Source: CAD feature listing. Evaluate the final solid. Frame: model axes, mm. A direction names the side the tool comes from. Give positions to 0.01 mm unless a question says otherwise; leave off trailing zeros. Order: outer loops, then holes, each group sorted by start corner. A loop starts at its lowest first (then second) coordinate and runs counter-clockwise, first axis right, second up. Notation, with made-up numbers: M -13,-9 L 3,-9 A23 cw 3,22 Z; hole C 62.25,-0.5 d5. An arc over 180 degrees is marked long. Answer as a JSON object with one key per item and string values. Group by question number.
1. Section query A-A (y = 76). Output: boundary loops of the cut face in (x, z).
2. Pin query (flat end, axial travel): P1, Ø10, axis at x = 19.05, z = -224.79, coming from the +Y side. Return the tip coordinate at first contact, or that it passes through.
3. Set-up query: faces 5 (the flat face through (38.1, 44, -222)), 6 (the flat face through (19, 44.45, -225)). Return all of +Z, -Z, +X, -X, +Y, -Y with unobstructed straight access to the full face (end or side cutting, diameter ignored); none if empty.
4. Section query B-B (x = 9.5). Output: boundary loops of the cut face in (y, z).
5. Section query C-C (z = -232.5). Output: boundary loops of the cut face in (x, y).
6. Pull-direction query (Z, two-part tool) for faces 1 (the flat face through (23, 0, -228)), 2 (the flat face through (19, 44, 0)), 3 (the flat face through (19, 67, -243.84)), 4 (the flat face through (19, 67, -205.74)); classes: +Z half, -Z half, draft (parallel to the pull), parting line (faces both ways), or undercut.
7. Material intervals for L1, parallel to X at y = 4.25, z = -224.79 (3 decimals); L2, parallel to Z at x = 16, y = 47; L3, parallel to Z at x = 19.05, y = 6.5 (3 decimals), sorted ascending. Write a range as [from, to].
Autodesk Inventor part; units mm, degrees
ref_plane "YZ Plane" through (0, 0, 0) normal (1, 0, 0) x (0, 1, 0)
ref_plane "XZ Plane" through (0, 0, 0) normal (0, 1, 0) x (-1, 0, 0)
ref_plane "XY Plane" through (0, 0, 0) normal (0, 0, 1) x (1, 0, 0)
sketch "Sketch1" plane through (0, 0, 0) normal (1, 0, 0) x (0, 1, 0)
  line L0 (0, 0) -> (88.9, 0)
  line L1 (88.9, 0) -> (88.9, -449.58)
  line L2 (88.9, -449.58) -> (0, -449.58)
  line L3 (0, -449.58) -> (0, 0)
  dimension "d0" = 88.9
  dimension "d1" = 449.58
extrude "Extrusion1" add sketch "Sketch1" along normal blind 38.1
sketch "Sketch2" plane through (38.1, 0, 0) normal (1, 0, 0) x (0, 0, -1)
  line L0 (0, 88.9) -> (0, 0)
  line L1 (0, 0) -> (449.58, 0)
  line L2 (449.58, 88.9) -> (0, 88.9)
  line L3 (205.74, 88.9) -> (205.74, 44.45)
  line L4 (224.79, 88.9) -> (224.79, 0) construction
  line L5 (243.84, 88.9) -> (243.84, 44.45)
  line L6 (205.74, 44.45) -> (243.84, 44.45)
  line L7 (205.74, 88.9) -> (243.84, 88.9)
  dimension "d4" = 44.45
  dimension "d5" = 205.74
extrude "Extrusion2" cut sketch "Sketch2" against normal blind 50.8
sketch "Sketch3" plane through (0, 0, -449.58) normal (0, -1, 0) x (1, 0, 0)
  line L0 (0, 0) -> (0, 449.58)
  line L1 (0, 0) -> (38.1, 0)
  line L2 (38.1, 449.58) -> (38.1, 0)
  line L3 (0, 449.58) -> (38.1, 449.58)
  line L4 (19.05, 449.58) -> (19.05, 0) construction
  line L5 (0, 224.79) -> (38.1, 224.79) construction
  circle A0 centre (19.05, 224.79) radius 7.9481
hole "Hole1" at (19.05, 0, -224.79) direction (0, 1, 0) diameter 6.35 depth 12.7 tip angle 118
properties part number "hubRingInnerWood" material "Wood (Oak)"
Answer sheet:
{
 "1": {"outline": "M 0,-449.58 L 38.1,-449.58 L 38.1,-243.84 L 0,-243.84 Z; M 0,-205.74 L 38.1,-205.74 L 38.1,0 L 0,0 Z"},
 "2": {"P1": "y = 44.45"},
 "3": {"face 5": "+Z, -Z, +X, +Y, -Y", "face 6": "+X, -X, +Y"},
 "4": {"outline": "M 0,-449.58 L 88.9,-449.58 L 88.9,-243.84 L 44.45,-243.84 L 44.45,-205.74 L 88.9,-205.74 L 88.9,0 L 0,0 Z"},
 "5": {"outline": "M 0,0 L 38.1,0 L 38.1,44.45 L 0,44.45 Z"},
 "6": {"face 1": "draft", "face 2": "+Z half", "face 3": "undercut", "face 4": "undercut"},
 "7": {"L1": "[0, 15.875], [22.225, 38.1]", "L2": "[-449.58, -243.84], [-205.74, 0]", "L3": "[-449.58, -227.965], [-221.615, 0]"}
}
